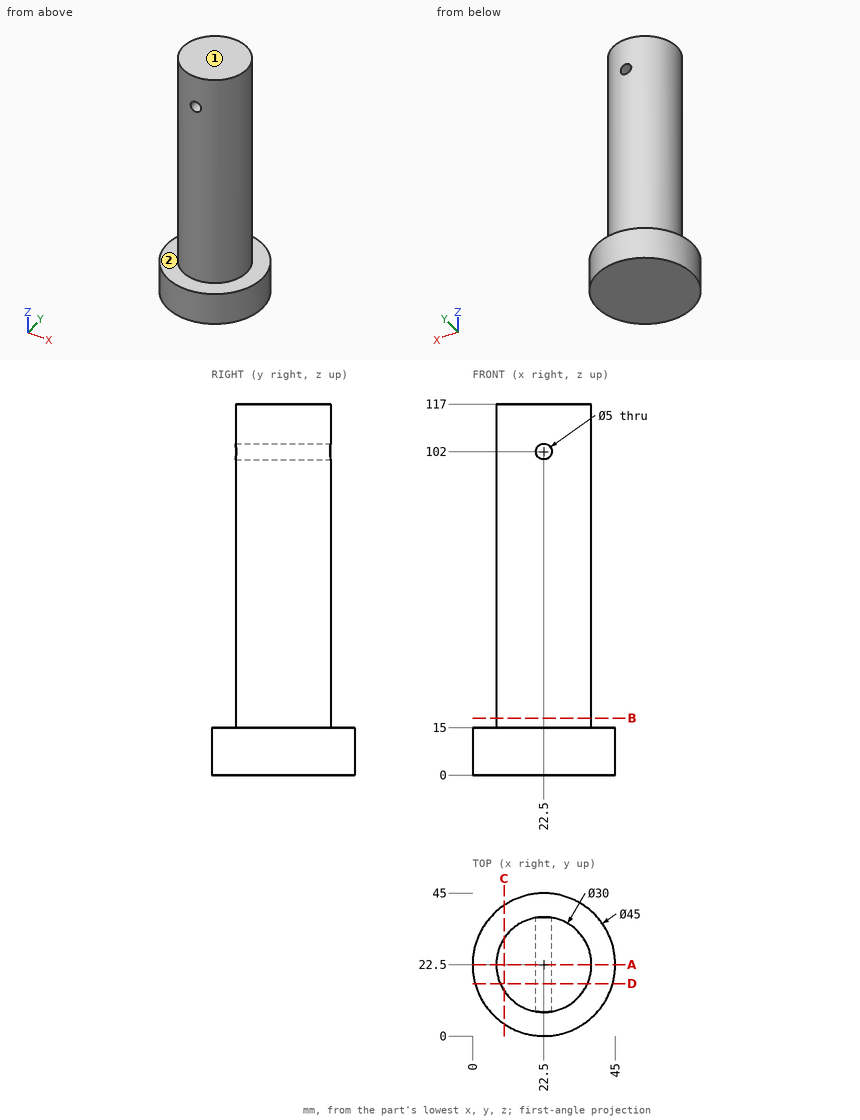
Design review of the part shown in the three views and the two pictorial views. Dimensions are in mm from the part's minimum x, y and z. A direction names the side the tool comes from. Give positions to 0.01 mm unless a question says otherwise; leave off trailing zeros. Write each loop counter-clockwise with the first axis right and the second up, starting at its lowest first coordinate (ties: lowest second). Pieces come first, ordered by that corner, then holes. Notation, with made-up numbers: M 59.5,76.25 L 117.5,76.25 A25 cw 117.5,100.25 Z; hole C 60,3 d2. An arc over 180 degrees is marked long. Answer as CSV lines item,"result".
1. Consider section D-D, the plane y = 16.5. Write out the cut boundary in (x, z), then the cut area to 3 significant figures.
Findings:
outline,"M 0.81,0 L 44.19,0 L 44.19,15 L 36.25,15 L 36.25,117 L 8.75,117 L 8.75,15 L 0.81,15 Z; hole C 22.5,102 d5"
area,"3,440 mm2"
2. Consider section C-C, the plane x = 10. Write out the cut boundary in (y, z).
Findings:
outline,"M 3.79,0 L 41.21,0 L 41.21,15 L 30.79,15 L 30.79,117 L 14.21,117 L 14.21,15 L 3.79,15 Z"
3. For pin 1 (4 mm diameter, centred on x = 14.5, z = 67.5, fed in from +Y); pin 2 (6 mm diameter, centred on y = 6, z = 102, fed in from -X); pin 3 (4 mm diameter, centred on y = 31, z = 93, fed in from +X), all flat-tipped, find the tip position at first contact; note any pin that passes through.
Findings:
pin 1,"stops at y = 36.25"
pin 2,"stops at x = 15.96"
pin 3,"stops at x = 36.02"
4. For the marked faces 1 and 2, list the 3-axis set-ups (+Z, -Z, +X, -X, +Y, -Y) from which the entire face can be reached by the end or side of a thin tool; tool diameter is ignored.
Findings:
face 1,"+Z, +X, -X, +Y, -Y"
face 2,"+Z"
5. Consider section A-A, the plane y = 22.5. Write out the cut boundary in (x, z), then the cut area to 3 significant figures.
Findings:
outline,"M 0,0 L 45,0 L 45,15 L 37.5,15 L 37.5,117 L 7.5,117 L 7.5,15 L 0,15 Z; hole C 22.5,102 d5"
area,"3,720 mm2"
6. Wall thickness on line 1 (Z direction, x = 22.5, y = 29.5); line 2 (Z direction, x = 28, y = 3); line 3 (X direction, y = 17, z = 102): over which ranges is each line inside the solid? List them lowest first.
Findings:
line 1,"z = 0 to 99.5, 104.5 to 117"
line 2,"z = 0 to 15"
line 3,"x = 8.54 to 20, 25 to 36.46"
7. Consider section B-B, the plane z = 18. Write out the cut boundary in (x, y), then the cut area to 3 significant figures.
Findings:
outline,"C 22.5,22.5 d30"
area,"707 mm2"
